Here's how the part is built. I have some questions about the finished solid (model axes, mm). Face numbers are marked on the shaded views. A direction names the side the tool comes from. Coordinates: 2 decimals unless noted, no trailing zeros. Write each loop counter-clockwise with the first axis right and the second up, starting at its lowest first coordinate (ties: lowest second). Pieces come first, ordered by that corner, then holes. Notation, with made-up numbers: M 47,88 L 54,88 A32 ccw 54,121 Z; hole C 57.25,54 d8. An arc over 180 degrees is marked long. Use a Markdown table: item, result.
```python
from build123d import *

# Parameters (mm, degrees)
EXTRUDE_1_DEPTH = 20
EXTRUDE_1_TAPER = 5
SKETCH_2_R      = 40
EXTRUDE_2_DEPTH = 4
SKETCH_3_R      = 21
EXTRUDE_3_DEPTH = 109
CHAMFER_1_SIZE  = 2
CHAMFER_2_SIZE  = 2
EXTRUDE_5_DEPTH = 160
SKETCH_7_W      = 50
SKETCH_7_H      = 80
EXTRUDE_6_DEPTH = 50
EXTRUDE_7_DEPTH = 40


with BuildPart() as part:
    # 草圖1 → 伸長1 (new body)
    with BuildSketch(Plane(origin=(0, 0, 0), x_dir=(0, 0, -1), z_dir=(1, 0, 0))):
        with BuildLine():
            ThreePointArc((-34, 54), (-48.142135624, 48.142135624), (-54, 34))
            Line((-54, 34), (-54, -34))
            ThreePointArc((-54, -34), (-48.142135624, -48.142135624), (-34, -54))
            Line((-34, -54), (34, -54))
            ThreePointArc((34, -54), (48.142135624, -48.142135624), (54, -34))
            Line((54, -34), (54, 34))
            ThreePointArc((54, 34), (48.142135624, 48.142135624), (34, 54))
            Line((34, 54), (-34, 54))
        make_face()
    extrude(amount=EXTRUDE_1_DEPTH, taper=EXTRUDE_1_TAPER)

    # 草圖2 → 伸長2 (add)
    with BuildSketch(Plane(origin=(20, 0, 0), x_dir=(0, 0, -1), z_dir=(1, 0, 0))):
        Circle(SKETCH_2_R)
    extrude(amount=EXTRUDE_2_DEPTH)

    # 草圖3 → 伸長3 (add)
    with BuildSketch(Plane(origin=(24, 0, 0), x_dir=(0, 0, -1), z_dir=(1, 0, 0))):
        Circle(SKETCH_3_R)
    extrude(amount=EXTRUDE_3_DEPTH)

    # 導角1
    chamfer_1_edges = [part.edges().sort_by_distance(p)[0] for p in [
        (24, 0, 21),
    ]]
    chamfer(chamfer_1_edges, length=CHAMFER_1_SIZE)

    # 導角2
    chamfer_2_edges = [part.edges().sort_by_distance(p)[0] for p in [
        (133, 0, 21),
    ]]
    chamfer(chamfer_2_edges, length=CHAMFER_2_SIZE)

    # 草圖6 → 伸長5 (add)
    with BuildSketch(Plane.ZY):
        with BuildLine():
            Line((-54, 34), (-54, -34))
            ThreePointArc((-54, -34), (-48.142135624, -48.142135624), (-34, -54))
            Line((-34, -54), (34, -54))
            ThreePointArc((34, -54), (48.142135624, -48.142135624), (54, -34))
            Line((54, -34), (54, 34))
            ThreePointArc((54, 34), (48.142135624, 48.142135624), (34, 54))
            Line((34, 54), (-34, 54))
            ThreePointArc((-34, 54), (-48.142135624, 48.142135624), (-54, 34))
        make_face()
    extrude(amount=EXTRUDE_5_DEPTH)

    # 草圖7 → 伸長6 (add)
    with BuildSketch(Plane(origin=(0, 54, 0), x_dir=(1, 0, 0), z_dir=(0, 1, 0))):
        with Locations((-75, 0)):
            Rectangle(SKETCH_7_W, SKETCH_7_H)
    extrude(amount=EXTRUDE_6_DEPTH)

    # 草圖8 → 伸長7 (add)
    with BuildSketch(Plane.ZY.offset(160)):
        with BuildLine():
            Line((-53, 34), (-53, -34))
            ThreePointArc((-53, -34), (-47.435028843, -47.435028843), (-34, -53))
            Line((-34, -53), (34, -53))
            ThreePointArc((34, -53), (47.435028843, -47.435028843), (53, -34))
            Line((53, -34), (53, 34))
            ThreePointArc((53, 34), (47.435028843, 47.435028843), (34, 53))
            Line((34, 53), (-34, 53))
            ThreePointArc((-34, 53), (-47.435028843, 47.435028843), (-53, 34))
        make_face()
    extrude(amount=EXTRUDE_7_DEPTH)


solid = part.part
```
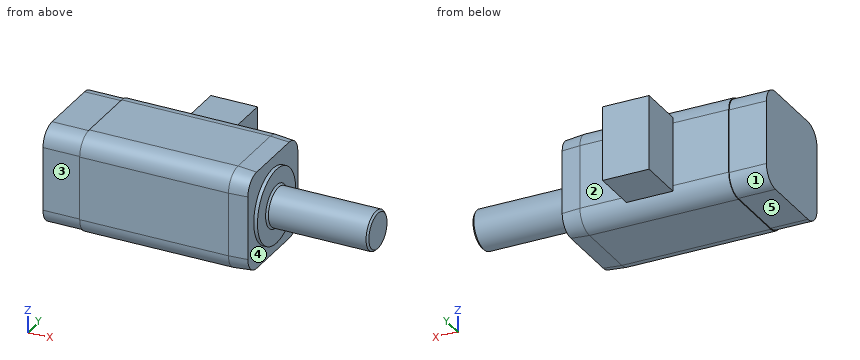
1. Suppose I cut it at A-A on x = -62. Write out the boundary of the cut face in (y, z), and give its area (3 significant figures).
Answers follow:
| item | result |
|---|---|
| outline | M -54,-34 A20 ccw -34,-54 L 34,-54 A20 ccw 54,-34 L 54,-40 L 104,-40 L 104,40 L 54,40 L 54,34 A20 ccw 34,54 L -34,54 A20 ccw -54,34 Z |
| area | 15,300 mm2 |
2. I need wall thicknesses on probe 1 along Z at (x, y) = (-71, 64); probe 2 along X at (y, z) = (-11, -15.5); probe 3 along X at (y, z) = (-28, 47). Which ranges of each line are inside material? Lowest first, please.
Answers follow:
| item | result |
|---|---|
| probe 1 | z = -40 to 40 |
| probe 2 | x = -200 to 132.99 |
| probe 3 | x = -200 to 20 |
3. Which directions (+Z, -Z, +X, -X, +Y, -Y) give clear straight access to the entire face, cutting with the end or side of a thin tool? Please do the marked faces 1, 2, 3, 4 and 5.
Answers follow:
| item | result |
|---|---|
| face 1 | -Z, -X, +Y |
| face 2 | +Z, -Z, +X, +Y |
| face 3 | +Z, -Z, -X, -Y |
| face 4 | +X |
| face 5 | -Z, -X, +Y, -Y |
4. Suppose I cut it at C-C on x = 88.5. Write out the boundary of the cut face in (y, z).
Answers follow:
| item | result |
|---|---|
| outline | C 0,0 d42 |
5. Suppose I cut it at B-B on y = 74. Write out the boundary of the cut face in (x, z), and give its area (3 significant figures).
Answers follow:
| item | result |
|---|---|
| outline | M -100,-40 L -50,-40 L -50,40 L -100,40 Z |
| area | 4,000 mm2 |
6. Will these pins go through, and if not, where does the flat tip stop? pin 1 Ø12 at (x, z) = (-184.5, -7.5) entering from +Y; pin 2 Ø5 at (x, z) = (-76.5, -38) entering from -Y; pin 3 Ø1 at (x, z) = (19.5, 43) entering from +Y.
Answers follow:
| item | result |
|---|---|
| pin 1 | stops at y = 53 |
| pin 2 | stops at y = -53.94 |
| pin 3 | stops at y = 50.2 |
